```python
from build123d import *

# Parameters (mm, degrees)
SKETCH3_R             = 5
BOSS_EXTRUDE1_DEPTH   = 15
BOSS_EXTRUDE1_2_DEPTH = 15
BOSS_EXTRUDE1_3_DEPTH = 15
BOSS_EXTRUDE1_4_DEPTH = 15
SKETCH4_R             = 7.575
BOSS_EXTRUDE2_DEPTH   = 4
SKETCH5_R             = 12.5
BOSS_EXTRUDE3_DEPTH   = 4.5
SKETCH6_R             = 13
SKETCH6_R_2           = 12.5
BOSS_EXTRUDE4_DEPTH   = 0.5


with BuildPart() as part:
    # Sketch3 → Boss-Extrude1 (new body)
    with BuildSketch(Plane(origin=(0, 0, 19), x_dir=(-1, 0, 0), z_dir=(0, 0, -1))):
        with Locations((-11.313708499, 11.313708499)):
            Circle(SKETCH3_R)
    extrude(amount=BOSS_EXTRUDE1_DEPTH)



with BuildPart() as body_2:
    # Sketch3 → Boss-Extrude1 2 (new body)
    with BuildSketch(Plane(origin=(0, 0, 19), x_dir=(-1, 0, 0), z_dir=(0, 0, -1))):
        with Locations((11.313708499, 11.313708499)):
            Circle(SKETCH3_R)
    extrude(amount=BOSS_EXTRUDE1_2_DEPTH)


with BuildPart() as body_3:
    # Sketch3 → Boss-Extrude1 3 (new body)
    with BuildSketch(Plane(origin=(0, 0, 19), x_dir=(-1, 0, 0), z_dir=(0, 0, -1))):
        with Locations((11.313708499, -11.313708499)):
            Circle(SKETCH3_R)
    extrude(amount=BOSS_EXTRUDE1_3_DEPTH)


with BuildPart() as body_4:
    # Sketch3 → Boss-Extrude1 4 (new body)
    with BuildSketch(Plane(origin=(0, 0, 19), x_dir=(-1, 0, 0), z_dir=(0, 0, -1))):
        with Locations((-11.313708499, -11.313708499)):
            Circle(SKETCH3_R)
    extrude(amount=BOSS_EXTRUDE1_4_DEPTH)


with BuildPart() as part_1:
    add(part.part)

    add(body_2.part)  # Boss-Extrude2 merges body 2

    add(body_3.part)  # Boss-Extrude2 merges body 3

    add(body_4.part)  # Boss-Extrude2 merges body 4
    # Sketch4 → Boss-Extrude2 (add)
    with BuildSketch(Plane(origin=(0, 0, 19), x_dir=(-1, 0, 0), z_dir=(0, 0, -1))):
        with BuildLine():
            Line((16.313708499, -11.313708499), (16.313708499, 11.313708499))
            ThreePointArc((16.313708499, 11.313708499), (7.778174593, 7.778174593), (11.313708499, 16.313708499))
            Line((11.313708499, 16.313708499), (-11.313708499, 16.313708499))
            ThreePointArc((-11.313708499, 16.313708499), (-7.778174593, 14.849242405), (-6.313708499, 11.313708499))
            ThreePointArc((-6.313708499, 11.313708499), (-11.313708499, 6.313708499), (-16.313708499, 11.313708499))
            Line((-16.313708499, 11.313708499), (-16.313708499, -11.313708499))
            ThreePointArc((-16.313708499, -11.313708499), (-11.313708499, -6.313708499), (-6.313708499, -11.313708499))
            ThreePointArc((-6.313708499, -11.313708499), (-7.778174593, -14.849242405), (-11.313708499, -16.313708499))
            Line((-11.313708499, -16.313708499), (11.313708499, -16.313708499))
            ThreePointArc((11.313708499, -16.313708499), (7.778174593, -7.778174593), (16.313708499, -11.313708499))
        make_face()
        Circle(SKETCH4_R, mode=Mode.SUBTRACT)
    extrude(amount=BOSS_EXTRUDE2_DEPTH)

    # Sketch5 → Boss-Extrude3 (add)
    with BuildSketch(Plane.XY.offset(19)):
        with Locations(Location((0, 0, 0), (0, 0, 180))):
            Circle(SKETCH5_R)
    extrude(amount=BOSS_EXTRUDE3_DEPTH)

    # Sketch6 → Boss-Extrude4 (add)
    with BuildSketch(Plane.XY.offset(19)):
        with Locations(Location((0, 0, 0), (0, 0, 180))):
            Circle(SKETCH6_R)
        Circle(SKETCH6_R_2, mode=Mode.SUBTRACT)
    extrude(amount=BOSS_EXTRUDE4_DEPTH)


solid = part_1.part
```
Could you check a few things on this model? Use its own coordinates, in mm. A direction names the side the tool comes from. Round coordinates to 2 decimals unless told otherwise and drop trailing zeros. Order: outer loops, then holes, each group sorted by start corner. A loop starts at its lowest first (then second) coordinate and runs counter-clockwise, first axis right, second up. Notation, with made-up numbers: M -39.75,2.25 L 15.25,2.25 A23 ccw 15.25,32.25 Z; hole C -1,-35 d8. An arc over 180 degrees is marked long. One line per question, with ' | ' between items. Start each with the question number.
(1) For P1, Ø10, axis at x = 7, y = -5, coming from the -Z side; P2, Ø4, axis at y = 11, z = 21.5, coming from the +X side; P3, Ø4, axis at y = 3, z = 11, coming from the +X side; P4, Ø6, axis at x = -7.5, z = 11, coming from the +Y side, each with a flat end and sliding along its axis, tell me the tip position at first contact or that it passes through.
(2) Suppose I cut it at B-B on x = 0. List the corners of the cut face in (y, z) for me (3 decimals).
(3) Thinking about a two-plate mould opening in X: for faces 4 (the face through (10.316, 7.91, 19.246)), 5 (the face through (0, 0, 19)), 6 (the face through (-11, -11, 4)), which applies, +X half, -X half, draft (parallel to the pull), parting line (faces both ways), or undercut?
(4) Suppose I cut it at D-D on z = 7.25. List the corners of the cut face in (x, y) for me.
(5) Suppose I cut it at A-A on z = 17.25. List the corners of the cut face in (x, y) for me (3 decimals), then the cut area to 3 significant figures.
(6) Please list where these lines run through material, in increasing order: line 1 along Y through (x, z) = (0, 18.1) (3 decimals); line 2 along Z through (x, y) = (5.5, -10.5); line 3 along Z through (x, y) = (5, 1.5).
(7) For faces 1 (the face through (7.5, 11.1, 19)), 2 (the face through (12.398, -16.195, 9.938)), 3 (the face through (11, 11, 4)), which set-ups out of +Z, -Z, +X, -X, +Y, -Y let a thin tool reach every point of the face, with its end or its side?
Geometry results:
1) P1: z = 4 | P2: x = 8.67 | P3: through | P4: y = 16.25
2) outline: M -16.314,15 L -7.575,15 L -7.575,19 L 7.575,19 L 7.575,15 L 16.314,15 L 16.314,19 L 13,19 L 13,19.5 L 12.5,19.5 L 12.5,23.5 L -12.5,23.5 L -12.5,19.5 L -13,19.5 L -13,19 L -16.314,19 Z
3) face 4: parting line | face 5: undercut | face 6: draft
4) outline: C -11.31,-11.31 d10; C -11.31,11.31 d10; C 11.31,-11.31 d10; C 11.31,11.31 d10
5) outline: M -16.314,-11.314 A5 ccw -11.314,-16.314 L 11.314,-16.314 A5 ccw 16.314,-11.314 L 16.314,11.314 A5 ccw 11.314,16.314 L -11.314,16.314 A5 ccw -16.314,11.314 Z; hole C 0,0 d15.15 | area: 863 mm²
6) line 1: -16.314 to -7.575, 7.575 to 16.314 | line 2: 15 to 23.5 | line 3: 19 to 23.5
7) face 1: +Z | face 2: -Z | face 3: -Z, +X, -X, +Y, -Y
